```python
from build123d import *

# Parameters (mm, degrees)
SKETCH1_R           = 4.7
BOSS_EXTRUDE1_DEPTH = 60
CHAMFER1_SIZE       = 1
CHAMFER1_SIZE2      = 1.732050808
CHAMFER3_SIZE       = 1
CHAMFER3_SIZE2      = 1.732050808


with BuildPart() as part:
    # Sketch1 → Boss-Extrude1 (new body)
    with BuildSketch(Plane(origin=(0, 0, 0), x_dir=(1, 0, 0), z_dir=(0, 1, 0))):
        with Locations(Location((0, 0, 0), (0, 0, 270))):
            Circle(SKETCH1_R)
    extrude(amount=BOSS_EXTRUDE1_DEPTH)

    # Chamfer1
    chamfer1_edges = [part.edges().sort_by_distance(p)[0] for p in [
        (0, 0, -4.7),
    ]]
    chamfer1_side = [part.faces().sort_by_distance(p)[0] for p in [
        (0, 0, 0),
    ]]
    chamfer(chamfer1_edges, length=CHAMFER1_SIZE, length2=CHAMFER1_SIZE2, reference=chamfer1_side[0])

    # Chamfer3
    chamfer3_edges = [part.edges().sort_by_distance(p)[0] for p in [
        (0, 60, -4.7),
    ]]
    chamfer3_side = [part.faces().sort_by_distance(p)[0] for p in [
        (0, 60, 0),
    ]]
    chamfer(chamfer3_edges, length=CHAMFER3_SIZE, length2=CHAMFER3_SIZE2, reference=chamfer3_side[0])


solid = part.part
```
Input: part model. Units: mm. Frame: model coordinates. Give positions to 0.01 mm unless a question says otherwise; leave off trailing zeros. Loops run counter-clockwise (first coordinate to the right, second up) from the corner with the lowest first, then second, coordinate; pieces in that order, holes last.
1) Section query A-A on y = 55.5. Return the cut outline in (x, z), and give its area (3 significant figures).
A:
outline: circle Ø9.4 at (0, 0)
area: 69.4 mm2
2) Contact query for flat-ended pins moving along their axis: pin 1 (5 mm diameter, centred on y = 42.5, z = -3.5, fed in from -X); pin 2 (4 mm diameter, centred on y = 38, z = -2.5, fed in from -X); pin 3 (1.5 mm diameter, centred on x = 3.5, y = 43, fed in from +Z). Output: stop coordinate, or through.
A:
pin 1: stops at x = -4.59
pin 2: stops at x = -4.67
pin 3: stops at z = 3.81
3) Line query: L1, parallel to X at y = 7.5, z = 0.25; L2, parallel to X at y = 33.5, z = -3.5; L3, parallel to Z at x = -1, y = 45. Output: solid intervals per line, ascending.
A:
L1: x = -4.69 to 4.69
L2: x = -3.14 to 3.14
L3: z = -4.59 to 4.59
